The model under review builds one solid part; all positions refer to its coordinate system, in mm. Face numbers are marked on the shaded views. A direction names the side the tool comes from. Coordinates: 2 decimals unless noted, no trailing zeros. Loops run counter-clockwise (first coordinate to the right, second up) from the corner with the lowest first, then second, coordinate; pieces in that order, holes last. Notation, with made-up numbers: M 18.25,27.5 L 34.25,27.5 A15 cw 34.25,31.5 Z; hole C 71,81 d6. An arc over 180 degrees is marked long. One line per item, written item: value.
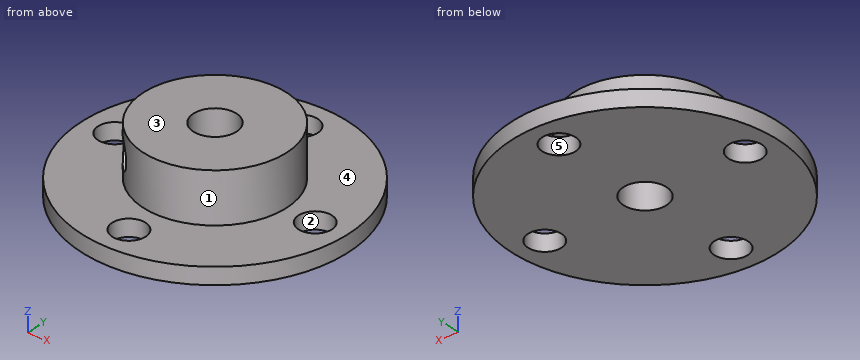
```python
from build123d import *

# Parameters (mm, degrees)
F_1_8_0_125_DIAMETER_HOLE1_D = 3.175
F_6_32_TAPPED_HOLE1_D        = 2.7051
F_6_32_TAPPED_HOLE1_DEPTH    = 6.858
F_6_32_TAPPED_HOLE1_TIP      = 0.81269403


with BuildPart() as part:
    # Sketch1 → Revolve1 (revolve)
    with BuildSketch(Plane(origin=(15.304322218, 0, 0), x_dir=(0, 0, -1), z_dir=(1, 0, 0)), mode=Mode.PRIVATE) as revolve1_sk:
        Polygon((-7.493, 22.653467802), (-7.493, 12.003467802), (-9.0805, 12.003467802), (-9.0805, 17.890967802), (-13.843, 17.890967802), (-13.843, 22.653467802), align=None)
    revolve(revolve1_sk.sketch.rotate(Axis((15.304322218, 24.703467802, 13.843), (0, 0, -1)), 270), axis=Axis((15.304322218, 24.703467802, 13.843), (0, 0, -1)))

    # 1/8 (0.125) Diameter Hole1 (through all)
    with Locations(Plane.XY.offset(9.0805)):
        with Locations((15.304322218, 14.947217802), (25.060572218, 24.703467802), (15.304322218, 34.459717802), (5.548072218, 24.703467802)):
            Hole(F_1_8_0_125_DIAMETER_HOLE1_D / 2)

    # #6-32 Tapped Hole1
    with Locations(Plane(origin=(15.186730063, 15.186730063, 0), x_dir=(0, 0, 1), z_dir=(-0.7071067811865488, -0.7071067811865464, 0))):
        with Locations((11.46175, 6.646199579)):
            Hole(F_6_32_TAPPED_HOLE1_D / 2, depth=F_6_32_TAPPED_HOLE1_DEPTH)
            with Locations((0, 0, -(F_6_32_TAPPED_HOLE1_DEPTH + F_6_32_TAPPED_HOLE1_TIP / 2))):  # 118° drill point
                Cone(0, F_6_32_TAPPED_HOLE1_D / 2, F_6_32_TAPPED_HOLE1_TIP, mode=Mode.SUBTRACT)


solid = part.part
```
(1) To check wall thickness, follow L1, parallel to X at y = 24.75, z = 13.25; L2, parallel to Z at x = 10, y = 17; L3, parallel to Y at x = 16.75, z = 11.5. State the ranges of each line that lie inside material, in increasing order. Write a range as [from, to].
Checks:
L1: [8.49, 13.25], [17.35, 22.12]
L2: [7.49, 9.08]
L3: [18.05, 23.25], [26.16, 31.36]
(2) Add section D-D on y = 29. State the section outline as (x, z) points, then the cut area to 3 significant figures.
Checks:
outline: M 3.35,7.49 L 27.26,7.49 L 27.26,9.08 L 20.59,9.08 L 20.59,13.84 L 10.02,13.84 L 10.02,9.08 L 3.35,9.08 Z
area: 88.3 mm^2
(3) Tool access review of the marked faces 4 and 5: name each direction out of +Z, -Z, +X, -X, +Y, -Y from which nothing blocks a thin tool from reaching the whole face with its end or side.
Checks:
face 4: +Z
face 5: +Z, -Z
(4) Add section A-A on x = 24.25. State the section outline as (y, z) points.
Checks:
outline: M 15.69,7.49 L 23.34,7.49 L 23.34,9.08 L 15.69,9.08 Z; M 26.07,7.49 L 33.72,7.49 L 33.72,9.08 L 26.07,9.08 Z
(5) Insertion check: pin 1 Ø3.5 at (x, y) = (15.3, 14.95) entering from +Z; pin 2 Ø1.9 at (x, y) = (25.06, 24.7) entering from -Z; pin 3 Ø1 at (x, z) = (15, 10) entering from -Y; pin 4 Ø1 at (x, z) = (11, 8.5) entering from +Y. Each pin has a flat end and moves straight along its axis. Give the tip position at first contact, or say it passes through.
Checks:
pin 1: z = 9.08
pin 2: through
pin 3: y = 17.89
pin 4: y = 36.82
(6) Add section B-B on y = 14.25. State the section outline as (x, z) points.
Checks:
outline: M 8.09,7.49 L 13.88,7.49 L 13.88,9.08 L 8.09,9.08 Z; M 16.73,7.49 L 22.52,7.49 L 22.52,9.08 L 16.73,9.08 Z
(7) Draft analysis for pull direction X (two halves, no side actions). For the marked faces 1, 2 and 3, state which applies: pulls with the +X half, pulls with the -X half, needs draft (parallel to the pull), parting line crosses it, or undercut.
Checks:
face 1: parting line crosses it
face 2: undercut
face 3: needs draft
(8) Add section C-C on z = 8. State how many separate pieces and enclosed holes the cut face has, then the cut area to 3 significant figures.
Checks:
separate pieces: 1
enclosed holes: 5
area: 462 mm^2
